Verification items for the finished model (mm, model axes). A direction names the side the tool comes from. Round coordinates to 2 decimals unless told otherwise and drop trailing zeros. Write each loop counter-clockwise with the first axis right and the second up, starting at its lowest first coordinate (ties: lowest second). Pieces come first, ordered by that corner, then holes. Notation, with made-up numbers: M 3.5,-4 L 34.5,-4 A3 ccw 34.5,1 Z; hole C -39.75,25 d5. An arc over 180 degrees is marked long. Answer in a Markdown table with one row per item. Add a question column.
1. Sectioned sample at D-D on y = -37. Record the cut outline in (x, z).
2. Sectioned sample at A-A on x = 0. Record the cut outline in (y, z), plus the area to 3 significant figures.
3. Set-up check for faces 4 (the flat face through (13.33, -30, 15.13)), 5 (the flat face through (60, -20, -10)), 6 (the flat face through (0, -5, 0)), 7 (the flat face through (60, -20, 10)): record each of +Z, -Z, +X, -X, +Y, -Y from which the full face is reachable in a straight line by a thin tool's end or side.
4. Material ranges on probe 1 along Z at (x, y) = (0, -15); probe 2 along Z at (x, y) = (22, -19.5); probe 3 along Z at (x, y) = (57, -13), recorded low to high.
5. Sectioned sample at B-B on z = 0. Record the cut outline in (x, y).
6. Go/stop test with flat-tipped pins: pin 1 Ø12 at (x, z) = (48.5, 9) entering from +Y; pin 2 Ø16 at (x, y) = (57, -17) entering from -Z; pin 3 Ø4.5 at (x, z) = (0, 26.5) entering from -Y; pin 4 Ø1 at (y, z) = (-7.5, 16) entering from +X. Record where each tip stops, or that it passes through.
7. Sectioned sample at C-C on x = 71. Record the cut outline in (y, z).
8. Draft check along Z on faces 1 (the cylindrical face through (34.256, -14.79, -12.366)), 2 (the cylindrical face through (-0.234, -15.21, -24.715)), 3 (the cylindrical face through (34.256, -15.21, 12.366)). Enter one of: pulls with the +Z half, pulls with the -Z half, needs draft (parallel to the pull), parting line crosses it, or undercut.
```python
from build123d import *

# Parameters (mm, degrees)
F0_R           = 33
F1_DEPTH       = 5
F2_R           = 33
F2_R_2         = 20
F3_DEPTH       = 25
F4_R           = 1.8
F5_DEPTH       = 30.001
F7_W           = 20
F7_H           = 20
F8_DEPTH       = 52
F9_W           = 52
F9_H           = 20
F12_DEPTH      = 10
F11_R          = 5
F13_DEPTH      = 12.001
F13_DEPTH_BACK = 10
F14_R          = 20
F15_W          = 20
F15_H          = 20
F16_DEPTH      = 11
F17_R          = 1.7
F18_DEPTH      = 41.0010001
F19_W          = 17.3078954501
F19_H          = 20
F20_DEPTH      = 11
F21_R          = 1.7
F22_DEPTH      = 41.0010001
F23_W          = 5
F23_H          = 20
F24_DEPTH      = 41.0010001


# Not quite as in the source:
# - a feature names something its author has since deleted; it is built from what else it names


with BuildPart() as f1:
    # F0 (on Front) → F1 (new body)
    with BuildSketch(Plane.XZ):
        Circle(F0_R)
    extrude(amount=F1_DEPTH)

    # F2 (on face) → F3 (join)
    with BuildSketch(Plane.XZ.offset(5)):
        Circle(F2_R)
        Circle(F2_R_2, mode=Mode.SUBTRACT)
    extrude(amount=F3_DEPTH)

    # F4 (on face) → F5 (cut, through all)
    with BuildSketch(Plane.XZ.offset(30)):
        with Locations((0, 26.5)):
            Circle(F4_R)
        with Locations((22, 14.7732867027)):
            Circle(F4_R)
        with Locations((-22, 14.7732867027)):
            Circle(F4_R)
        with Locations((0, -26.5)):
            Circle(F4_R)
        with Locations((-22, -14.7732867027)):
            Circle(F4_R)
        with Locations((22, -14.7732867027)):
            Circle(F4_R)
    extrude(amount=-F5_DEPTH, mode=Mode.SUBTRACT)

    # F7 (on offset) → F8 (join)
    with BuildSketch(Plane.YZ.offset(29)):
        with Locations((-10, 0)):
            Rectangle(F7_W, F7_H)
    extrude(amount=F8_DEPTH)

    # F9 (on face) → F12 (join)
    with BuildSketch(Plane.XZ.offset(20)):
        with Locations((55, 0)):
            Rectangle(F9_W, F9_H)
    extrude(amount=F12_DEPTH)

    # F11 (on offset) → F13 (cut, two sides)
    with BuildSketch(Plane.YZ.offset(-21)) as f13_sk:
        with Locations((-15, 0)):
            Circle(F11_R)
    extrude(amount=-F13_DEPTH, mode=Mode.SUBTRACT)
    extrude(f13_sk.sketch, amount=F13_DEPTH_BACK, mode=Mode.SUBTRACT)

    # F14
    f14_edges = [f1.edges().sort_by_distance(p)[0] for p in [
        (31.44837, -15, -10),
        (31.44837, -15, 10),
    ]]
    fillet(f14_edges, radius=F14_R)

    # F15 (on face) → F16 (join)
    with BuildSketch(Plane.XZ.offset(30)):
        with Locations((71, 0)):
            Rectangle(F15_W, F15_H)
    extrude(amount=F16_DEPTH)

    # F17 (on face) → F18 (cut, through all)
    with BuildSketch(Plane.XZ.offset(41)):
        with Locations((71, 0)):
            Circle(F17_R)
    extrude(amount=-F18_DEPTH, mode=Mode.SUBTRACT)

    # F19 (on face) → F20 (join)
    with BuildSketch(Plane.XZ.offset(30)):
        with Locations((52.346052275, 0)):
            Rectangle(F19_W, F19_H)
    extrude(amount=F20_DEPTH)

    # F21 (on face) → F22 (cut, through all)
    with BuildSketch(Plane.XZ.offset(41)):
        with Locations((57.05, 0)):
            Circle(F21_R)
    extrude(amount=-F22_DEPTH, mode=Mode.SUBTRACT)

    # F23 (on face) → F24 (cut, through all)
    with BuildSketch(Plane.XZ.offset(41)):
        with Locations((78.5, 0)):
            Rectangle(F23_W, F23_H)
    extrude(amount=-F24_DEPTH, mode=Mode.SUBTRACT)


solid = f1.part
```
Geometry check:
| question | item | result |
|---|---|---|
| 1 | outline | M 43.69,-10 L 76,-10 L 76,10 L 43.69,10 Z; hole C 57.05,0 d3.4; hole C 71,0 d3.4 |
| 2 | outline | M -30,-33 L 0,-33 L 0,-28.3 L -30,-28.3 Z; M -30,-24.7 L 0,-24.7 L 0,24.7 L -30,24.7 L -30,20 L -5,20 L -5,-20 L -30,-20 Z; M -30,28.3 L 0,28.3 L 0,33 L -30,33 Z |
| 2 | area | 764 mm2 |
| 3 | face 4 | +Z, -Z, -X, -Y |
| 3 | face 5 | -Z, +X, +Y, -Y |
| 3 | face 6 | -Y |
| 3 | face 7 | +Z, +X, +Y, -Y |
| 4 | probe 1 | z = -33 to -28.3, -24.7 to -20, 20 to 24.7, 28.3 to 33 |
| 4 | probe 2 | z = -24.6 to -16.57, -12.97 to 12.97, 16.57 to 24.6 |
| 4 | probe 3 | z = -10 to -1.7, 1.7 to 10 |
| 5 | outline | M -33,-30 L -20,-30 L -20,-20 L -33,-20 Z; M -33,-10 L -20,-10 L -20,-5 L 20,-5 L 20,-30 L 43.69,-30 L 43.69,-41 L 55.35,-41 L 55.35,0 L -33,0 Z; M 58.75,-41 L 69.3,-41 L 69.3,0 L 58.75,0 Z; M 72.7,-41 L 76,-41 L 76,0 L 72.7,0 Z |
| 6 | pin 1 | stops at y = 0 |
| 6 | pin 2 | stops at z = -10 |
| 6 | pin 3 | stops at y = -30 |
| 6 | pin 4 | stops at x = 29.92 |
| 7 | outline | M -41,-10 L 0,-10 L 0,-1.7 L -41,-1.7 Z; M -41,1.7 L 0,1.7 L 0,10 L -41,10 Z |
| 8 | face 1 | pulls with the -Z half |
| 8 | face 2 | undercut |
| 8 | face 3 | pulls with the +Z half |
